from build123d import *

# Parameters (mm, degrees)
F0_R     = 1.5
F1_DEPTH = 3
F3_DEPTH = 8.9
F4_R     = 1.5
F5_DEPTH = 20
F6_R     = 1.5
F7_DEPTH = 3


with BuildPart() as f1:
    # F0 (on Front) → F1 (new body)
    with BuildSketch(Plane.XZ):
        with BuildLine():
            Line((5.9394528039, 2.640625), (2.9697264019, 9.3203125))
            ThreePointArc((2.9697264019, 9.3203125), (0, 11.25), (-2.9697264019, 9.3203125))
            Line((-2.9697264019, 9.3203125), (-5.9394528039, 2.640625))
            ThreePointArc((-5.9394528039, 2.640625), (0, -6.5), (5.9394528039, 2.640625))
        make_face()
        with Locations((0, 8)):
            Circle(F0_R, mode=Mode.SUBTRACT)
    extrude(amount=-F1_DEPTH)

    # F2 (on face) → F3 (join)
    with BuildSketch(Plane.XZ):
        with BuildLine():
            ThreePointArc((-2.0615528128, 4), (-2.3423292192, -3.8423292192), (4.5, 0))
            ThreePointArc((4.5, 0), (3.8423292192, 2.3423292192), (2.0615528128, 4))
            Line((2.0615528128, 4), (-2.0615528128, 4))
        make_face()
    extrude(amount=F3_DEPTH)

    # F4 (on face) → F5 (cut)
    with BuildSketch(Plane.XZ.offset(8.9)):
        Circle(F4_R)
    extrude(amount=-F5_DEPTH, mode=Mode.SUBTRACT)

    # F6 (on face) → F7 (join)
    with BuildSketch(Plane.XZ.offset(8.9)):
        with BuildLine():
            Line((-5.9394528039, -2.640625), (-2.9697264019, -9.3203125))
            ThreePointArc((-2.9697264019, -9.3203125), (0, -11.25), (2.9697264019, -9.3203125))
            Line((2.9697264019, -9.3203125), (5.9394528039, -2.640625))
            ThreePointArc((5.9394528039, -2.640625), (0, 6.5), (-5.9394528039, -2.640625))
        make_face()
        with Locations((0, -8)):
            Circle(F6_R, mode=Mode.SUBTRACT)
        with BuildLine():
            Line((-2.0615528128, 4), (2.0615528128, 4))
            ThreePointArc((2.0615528128, 4), (3.8423292192, 2.3423292192), (4.5, 0))
            ThreePointArc((4.5, 0), (-2.3423292192, -3.8423292192), (-2.0615528128, 4))
        make_face(mode=Mode.SUBTRACT)
        with BuildLine():
            ThreePointArc((4.5, 0), (3.8423292192, 2.3423292192), (2.0615528128, 4))
            Line((2.0615528128, 4), (-2.0615528128, 4))
            ThreePointArc((-2.0615528128, 4), (-2.3423292192, -3.8423292192), (4.5, 0))
        make_face()
        Circle(F6_R, mode=Mode.SUBTRACT)
    extrude(amount=F7_DEPTH)


solid = f1.part
Geometry: final body of the model. Coordinates: model frame, mm. A direction names the side the tool comes from. Coordinates: 2 decimals unless noted, no trailing zeros. Loops run counter-clockwise (first coordinate to the right, second up) from the corner with the lowest first, then second, coordinate; pieces in that order, holes last. Notation, with made-up numbers: (34, -30.5) - (91, -30.5) arc R15 ccw to (91, -26.5) - close; hole circle Ø2 at (56.5, -22). An arc over 180 degrees is marked (long way). One line per question, with ' | ' between items. Start each with the question number.
(1) Cut plane A-A on x = 0. Output: boundary loops of the cut face in (y, z).
(2) Ray query, L1, parallel to Z at x = 0, y = -10.25; L2, parallel to Y at x = 3.5, z = 3; L3, parallel to Z at x = 0, y = -5.5. Return the intervals inside material, ascending. Write a range as from..to.
(3) Draft query along Z for faces 1 (the cylindrical face through (-0.325, -10.379, -9.464)), 2 (the flat face through (4.475, 1.479, 5.934)), 3 (the flat face through (4.434, -10.379, -6.027)), 4 (the cylindrical face through (-0.325, 1.479, 6.536)). Return one class per face: +Z half, -Z half, draft (parallel to the pull), parting line (faces both ways), or undercut.
(4) Cut plane B-B on z = 5.25. Output: boundary loops of the cut face in (x, y), and give its area (3 significant figures).
(5) Cut plane C-C on y = 1.25. Output: boundary loops of the cut face in (x, z), and give its area (3 significant figures).
(6) First-contact query: pin 1 (2.5 mm diameter, centred on x = 0, z = -8, fed in from +Y) (1 decimal); pin 2 (2 mm diameter, centred on x = -0.5, y = -3, fed in from +Z); pin 3 (2 mm diameter, centred on x = -5, y = -5, fed in from -Z); pin 4 (2 mm diameter, centred on x = -2, y = -10, fed in from +Z). Flat tips, straight axial feed; report the tip coordinate or a pass-through.
(7) Reachability of faces 5 (the flat face through (-4.475, -10.379, -5.934)), 6 (the flat face through (0, -4, 4)), 7 (the cylindrical face through (0.181, -10.379, 6.497)), 8 (the cylindrical face through (-0.181, 1.479, -6.497)), 9 (the flat face through (3, -8.9, -4)) from +Z, -Z, +X, -X, +Y, -Y: full face, straight path, thin tool, end or side. Return the list, or none.
(8) Cut plane D-D on y = -4.5. Output: boundary loops of the cut face in (x, z), and give its area (3 significant figures).
Here are the results:
1) outline: (-11.9, -11.25) - (-8.9, -11.25) - (-8.9, -9.5) - (-11.9, -9.5) - close; (-11.9, -6.5) - (-8.9, -6.5) - (-8.9, -4.5) - (0, -4.5) - (0, -6.5) - (3, -6.5) - (3, -1.5) - (-11.9, -1.5) - close; (-11.9, 1.5) - (3, 1.5) - (3, 6.5) - (0, 6.5) - (0, 4) - (-8.9, 4) - (-8.9, 6.5) - (-11.9, 6.5) - close; (0, 9.5) - (3, 9.5) - (3, 11.25) - (0, 11.25) - close
2) L1: -11.25..-9.5, -6.5..-1.5, 1.5..6.5 | L2: -11.9..-8.9, 0..3 | L3: -4.5..-1.5, 1.5..4
3) face 1: undercut | face 2: +Z half | face 3: -Z half | face 4: undercut
4) outline: (-4.78, 0) - (4.78, 0) - (4.78, 3) - (-4.78, 3) - close; (-3.83, -11.9) - (3.83, -11.9) - (3.83, -8.9) - (-3.83, -8.9) - close | area: 51.7 mm²
5) outline: (-5.94, 2.64) arc R6.5 ccw (long way) to (5.94, 2.64) - (2.97, 9.32) arc R3.25 ccw to (-2.97, 9.32) - close; hole circle Ø3 at (0, 0); hole circle Ø3 at (0, 8) | area: 153 mm²
6) pin 1: through | pin 2: z = 4 | pin 3: z = -2.06 | pin 4: z = 6.42
7) face 5: -Z, -X, +Y, -Y | face 6: +Z, +X, -X | face 7: -Y | face 8: +Y | face 9: none
8) outline: (-2.06, 4) arc R4.5 ccw (long way) to (2.06, 4) - close; hole circle Ø3 at (0, 0) | area: 55.2 mm²
